```python
from build123d import *

# Parameters (mm, degrees)
BOX004_W     = 10
BOX004_H     = 40
BOX004_DEPTH = 100
BOX003_W     = 1.5
BOX003_H     = 53
BOX003_DEPTH = 80
BOX002_W     = 6.5
BOX002_H     = 57
BOX002_DEPTH = 57
FILLET002_R  = 2
FILLET003_R  = 4


with BuildPart() as slide_holder_central_hole:
    # Box004 → Box004 (new body)
    with BuildSketch(Plane(origin=(-2, 8.5, 8.5), x_dir=(1, 0, 0), z_dir=(0, 0, 1))):
        with Locations((5, 20)):
            Rectangle(BOX004_W, BOX004_H)
    extrude(amount=BOX004_DEPTH)


with BuildPart() as slide_holder_hole_fusion:
    # Box003 → Box003 (new body)
    with BuildSketch(Plane(origin=(2.5, 2, 2), x_dir=(1, 0, 0), z_dir=(0, 0, 1))):
        with Locations((0.75, 26.5)):
            Rectangle(BOX003_W, BOX003_H)
    extrude(amount=BOX003_DEPTH)

    # Fusion001: union slide holder central hole
    add(slide_holder_central_hole.part)


with BuildPart() as slider_holder_cut_fillet:
    # Box002 → Box002 (new body)
    with BuildSketch(Plane.XY):
        with Locations((3.25, 28.5)):
            Rectangle(BOX002_W, BOX002_H)
    extrude(amount=BOX002_DEPTH)

    # Fillet002
    fillet002_edges = [slider_holder_cut_fillet.edges().sort_by_distance(p)[0] for p in [
        (3.25, 0, 57),
        (3.25, 57, 57),
    ]]
    fillet(fillet002_edges, radius=FILLET002_R)

    # Cut002: cut slide holder hole fusion
    add(slide_holder_hole_fusion.part, mode=Mode.SUBTRACT)

    # Fillet003
    fillet003_edges = [slider_holder_cut_fillet.edges().sort_by_distance(p)[0] for p in [
        (1.25, 8.5, 57),
        (1.25, 48.5, 57),
        (5.25, 8.5, 57),
        (5.25, 48.5, 57),
    ]]
    fillet(fillet003_edges, radius=FILLET003_R)


solid = slider_holder_cut_fillet.part
```
Here's how the part is built. I have some questions about the finished solid (model axes, mm). A direction names the side the tool comes from. Round coordinates to 2 decimals unless told otherwise and drop trailing zeros. Order: outer loops, then holes, each group sorted by start corner. A loop starts at its lowest first (then second) coordinate and runs counter-clockwise, first axis right, second up. Notation, with made-up numbers: M -35.5,24 L 4.5,24 A7 cw 4.5,34 Z; hole C -25.5,53 d10. An arc over 180 degrees is marked long. Answer as CSV lines item,"result".
Item 1: Which directions (+Z, -Z, +X, -X, +Y, -Y) give clear straight access to the entire face, cutting with the end or side of a thin tool? Please do faces 5 (the flat face through (1, 29, 8.5)), 6 (the flat face through (4, 26, 7)), 7 (the flat face through (3, 57, 27)).
From the geometry:
face 5,"+Z, +X, -X"
face 6,"+Z"
face 7,"+Z, -Z, +X, -X, +Y"
Item 2: Please list where these lines run through material, in increasing order: L1, parallel to Y at x = 3.25, z = 31.5; L2, parallel to X at y = 28.5, z = 5; L3, parallel to Y at x = 4.5, z = 24. Write a range as [from, to].
From the geometry:
L1,"[0, 2], [55, 57]"
L2,"[0, 2.5], [4, 6.5]"
L3,"[0, 8.5], [48.5, 57]"
Item 3: Imagine slicing it at A-A on z = 33.5. List the corners of the cut face in (x, y) for me.
From the geometry:
outline,"M 0,0 L 6.5,0 L 6.5,8.5 L 4,8.5 L 4,2 L 2.5,2 L 2.5,8.5 L 0,8.5 Z; M 0,48.5 L 2.5,48.5 L 2.5,55 L 4,55 L 4,48.5 L 6.5,48.5 L 6.5,57 L 0,57 Z"
Item 4: Imagine slicing it at C-C on y = 20. List the corners of the cut face in (x, z) for me.
From the geometry:
outline,"M 0,0 L 6.5,0 L 6.5,8.5 L 4,8.5 L 4,2 L 2.5,2 L 2.5,8.5 L 0,8.5 Z"
Item 5: We'd pull the mould along X, two halves only. Please class faces 1 (the flat face through (1, 54, 57)), 2 (the flat face through (3, 2, 29)), 3 (the flat face through (2.5, 26, 7)), 4 (the flat face through (6.5, 26, 7)): +X half, -X half, draft (parallel to the pull), parting line (faces both ways), or undercut.
From the geometry:
face 1,"draft"
face 2,"undercut"
face 3,"undercut"
face 4,"+X half"
Item 6: For pin 1 (2 mm diameter, centred on x = 5, y = 38, fed in from +Z), with a flat end and sliding along its axis, tell me the tip position at first contact or that it passes through.
From the geometry:
pin 1,"z = 8.5"
Item 7: Imagine slicing it at B-B on x = 4.75. List the corners of the cut face in (y, z) for me.
From the geometry:
outline,"M 0,0 L 57,0 L 57,55 A2 ccw 55,57 L 52.5,57 A4 ccw 48.5,53 L 48.5,8.5 L 8.5,8.5 L 8.5,53 A4 ccw 4.5,57 L 2,57 A2 ccw 0,55 Z"
